from build123d import *

# Parameters (mm, degrees)
F0_W     = 100
F0_H     = 200
F1_DEPTH = 2
F2_W     = 100
F2_H     = 3
F3_DEPTH = 100
F4_R     = 49.99999
F5_R     = 10
F6_DEPTH = 25
F5_R_2   = 1
F7_DEPTH = 25


# Not quite as in the source:
# - a fillet or chamfer is up to 0.001 mm smaller than in the source, because OpenCascade refuses the exact size


with BuildPart() as f1:
    # F0 (on Top) → F1 (new body)
    with BuildSketch(Plane.XY):
        Rectangle(F0_W, F0_H)
    extrude(amount=F1_DEPTH)

    # F2 (on face) → F3 (join)
    with BuildSketch(Plane.XY.offset(2)):
        with Locations((0, -98.5)):
            Rectangle(F2_W, F2_H)
    extrude(amount=F3_DEPTH)

    # F4 (radius 50 in the source; OpenCascade refuses exactly that, so slightly less here)
    f4_edges = [f1.edges().sort_by_distance(p)[0] for p in [
        (-50, -98.5, 102),
        (50, -98.5, 102),
    ]]
    fillet(f4_edges, radius=F4_R)

    # F5 (on face) → F6 (cut)
    with BuildSketch(Plane.XZ.offset(100)):
        with Locations((0, 61.5095198154)):
            Circle(F5_R)
    extrude(amount=-F6_DEPTH, mode=Mode.SUBTRACT)

    # F5 (on face) → F7 (cut)
    with BuildSketch(Plane.XZ.offset(100)):
        with Locations((0, 61.5095198154)):
            Circle(F5_R)
        with Locations((30, 61.5095198154)):
            Circle(F5_R_2)
        with Locations((-30, 61.5095198154)):
            Circle(F5_R_2)
    extrude(amount=-F7_DEPTH, mode=Mode.SUBTRACT)


solid = f1.part
Verification items for the finished model (mm, model axes). A direction names the side the tool comes from. Coordinates: 2 decimals unless noted, no trailing zeros. Order: outer loops, then holes, each group sorted by start corner. A loop starts at its lowest first (then second) coordinate and runs counter-clockwise, first axis right, second up. Notation, with made-up numbers: (-2.75, 82.5) -> (14.25, 82.5) arc R10 cw to (14.25, 89.5) -> close; hole circle Ø4 at (85, 82). An arc over 180 degrees is marked (long way). Use CSV: the item, a comma, the result in double quotes. Start each with the question number.
Q1. Section check A-A, the plane z = 65.5. Record the cut outline in (x, y), and give its area (3 significant figures).
Q2. Depth check by flat-ended pin: P1, Ø12, axis at x = 0, z = 61.51, coming from the +Y side; P2, Ø6, axis at x = -29, y = -34.5, coming from the +Z side; P3, Ø3, axis at x = -13.5, y = -31.5, coming from the -Z side; P4, Ø6, axis at x = 28, z = 84, coming from the +Y side. Enter the tip coordinate at first touch or a pass-through.
Q3. Draft check along Z on faces 3 (the flat face through (-50, 0, 1)), 4 (the flat face through (-1, 1, 0)), 5 (the cylindrical face through (-1.302, -98.521, 71.424)). Enter one of: +Z half, -Z half, draft (parallel to the pull), parting line (faces both ways), or undercut.
Q4. Section check C-C, the plane x = -33. Record the cut outline in (y, z).
Q5. Thickness scan on line 1 along Z through (x, y) = (-11.5, 15); line 2 along Y through (x, z) = (9.5, 86); line 3 along Z through (x, y) = (-30, -98.5). Record the ranges inside material, lowest first.
Q6. Tool access check on faces 1 (the flat face through (50, 0, 1)), 2 (the flat face through (-1, 3, 2)). Record the directions out of +Z, -Z, +X, -X, +Y, -Y that give a thin tool (end or side, any length) a straight path to the whole face; none if there is none.
Q7. Section check D-D, the plane z = 34.5. Record the cut outline in (x, y).
Q8. Section check B-B, the plane y = -29. Record the cut outline in (x, z).
Returned:
1,outline,"(-48.14, -100) -> (-9.17, -100) -> (-9.17, -97) -> (-48.14, -97) -> close; (9.17, -100) -> (48.14, -100) -> (48.14, -97) -> (9.17, -97) -> close"
1,area,"234 mm^2"
2,P1,"passes through"
2,P2,"stops at z = 2"
2,P3,"stops at z = 0"
2,P4,"stops at y = -97"
3,face 3,"draft"
3,face 4,"-Z half"
3,face 5,"undercut"
4,outline,"(-100, 0) -> (100, 0) -> (100, 2) -> (-97, 2) -> (-97, 89.56) -> (-100, 89.56) -> close"
5,line 1,"z = 0 to 2"
5,line 2,"y = -100 to -97"
5,line 3,"z = 0 to 60.51, 62.51 to 92"
6,face 1,"+Z, -Z, +X, +Y, -Y"
6,face 2,"+Z, +X, -X, +Y"
7,outline,"(-50, -100) -> (50, -100) -> (50, -97) -> (-50, -97) -> close"
8,outline,"(-50, 0) -> (50, 0) -> (50, 2) -> (-50, 2) -> close"
